Build history of the part. All positions in model axes, mm. Round coordinates to 2 decimals unless told otherwise and drop trailing zeros. Write each loop counter-clockwise with the first axis right and the second up, starting at its lowest first coordinate (ties: lowest second). Pieces come first, ordered by that corner, then holes. Notation, with made-up numbers: (12, 23.5) - (56, 23.5) arc R21 ccw to (56, 60.5) - close; hole circle Ø3 at (2.5, 30). An arc over 180 degrees is marked (long way). Answer as a JSON object with one key per item and string values. Group by question number.
Item 1: Two-plate mould, pull along Y, no slides. Class faces 1 (the flat face through (-127, -2, 3)), 2 (the flat face through (-2, 127, 3)), 3 (the cylindrical face through (-14.274, 0.628, 3.131)): +Y half, -Y half, draft (parallel to the pull), parting line (faces both ways), or undercut.
Item 2: Slice it at A-A, the plane y = 0. List the corners of the cut face in (x, z), then the cut area to 3 significant figures.
Item 3: Probe line 1 (Y direction, x = 0, z = 4.5); line 2 (Y direction, x = -97, z = 5.5); line 3 (X direction, y = 5, z = 1.5). List the from-to ranges inside material, lowest first. Write a range as from..to.
Item 4: Flat gauge pin, fed straight in: pin 1 (4 mm diameter, centred on x = -98.78, y = 98.78, fed in from +Z) (1 decimal). Where does the tip first touch, or does it go through?
from build123d import *

# Parameters (mm, degrees)
SKETCH1_W                      = 254
SKETCH1_H                      = 254
SKETCH1_R                      = 10.16
SKETCH1_R_2                    = 14.2875
BOSS_EXTRUDE2_DEPTH            = 6.35
F_9_0_196_DIAMETER_HOLE1_D     = 4.9784
F_9_0_196_DIAMETER_HOLE1_DEPTH = 6.35
F_9_0_196_DIAMETER_HOLE1_TIP   = 1.495662253


with BuildPart() as part:
    # Sketch1 → Boss-Extrude2 (new body)
    # profile 1 of 4: a face of its own
    with BuildSketch(Plane.XY):
        Rectangle(SKETCH1_W, SKETCH1_H)
        with Locations((-41.221968309, 29.688201844)):
            Circle(SKETCH1_R, mode=Mode.SUBTRACT)
        with Locations((0, 49.5808)):
            Circle(SKETCH1_R_2, mode=Mode.SUBTRACT)
        Circle(SKETCH1_R_2, mode=Mode.SUBTRACT)
        with Locations((41.221968309, 29.688201844)):
            Circle(SKETCH1_R, mode=Mode.SUBTRACT)
    # profile 2 of 4: a face of its own
    with BuildSketch(Plane.XY):
        with Locations((0, 49.5808)):
            Circle(SKETCH1_R_2)
    # profile 3 of 4: a face of its own
    with BuildSketch(Plane.XY):
        with Locations((41.221968309, 29.688201844)):
            Circle(SKETCH1_R)
    # profile 4 of 4: a face of its own
    with BuildSketch(Plane.XY):
        with Locations((-41.221968309, 29.688201844)):
            Circle(SKETCH1_R)
    extrude(amount=BOSS_EXTRUDE2_DEPTH)

    # #9 (0.196) Diameter Hole1
    with Locations(Plane(origin=(0, 0, 0), x_dir=(-1, 0, 0), z_dir=(0, 0, -1))):
        with Locations((-98.782817332, 98.782817332), (98.782817332, 98.782817332), (98.782817332, -98.782817332), (-98.782817332, -98.782817332)):
            Hole(F_9_0_196_DIAMETER_HOLE1_D / 2, depth=F_9_0_196_DIAMETER_HOLE1_DEPTH)
            with Locations((0, 0, -(F_9_0_196_DIAMETER_HOLE1_DEPTH + F_9_0_196_DIAMETER_HOLE1_TIP / 2))):  # 118° drill point
                Cone(0, F_9_0_196_DIAMETER_HOLE1_D / 2, F_9_0_196_DIAMETER_HOLE1_TIP, mode=Mode.SUBTRACT)


solid = part.part
Geometry says:
{
 "1": {"face 1": "draft", "face 2": "+Y half", "face 3": "undercut"},
 "2": {"outline": "(-127, 0) - (-14.29, 0) - (-14.29, 6.35) - (-127, 6.35) - close; (14.29, 0) - (127, 0) - (127, 6.35) - (14.29, 6.35) - close", "area": "1,430 mm^2"},
 "3": {"line 1": "y = -127..-14.29, 14.29..127", "line 2": "y = -127..-100.52, -97.05..97.05, 100.52..127", "line 3": "x = -127..-13.38, 13.38..127"},
 "4": {"pin 1": "passes through"}
}
